Can you work these out from the model? Positions are in its coordinate system, mm. A direction names the side the tool comes from. Give positions to 0.01 mm unless a question says otherwise; leave off trailing zeros. Loops run counter-clockwise (first coordinate to the right, second up) from the corner with the lowest first, then second, coordinate; pieces in that order, holes last. Notation, with made-up numbers: (36, 49) - (56, 49) arc R20 ccw to (56, 85) - close; hole circle Ø3 at (7, 66). An arc over 180 degrees is marked (long way). Write item = value, one per line.
from build123d import *

# Parameters (mm, degrees)
SKETCH_2_R          = 13
EXTRUDE_1_DEPTH     = 1.1
CUT_EXTRUDE_1_REACH = 21.053
SKETCH_3_R          = 7.5


with BuildPart() as part:
    # 草图1 → 旋转1 (revolve)
    with BuildSketch(Plane(origin=(0, 0, 0), x_dir=(-1, 0, 0), z_dir=(0, 0, -1)), mode=Mode.PRIVATE) as revolve_1_sk:
        with BuildLine():
            Line((-11.7, 0), (-7.8, 0))
            Line((-7.8, 0), (-7.5, 0))
            Line((-7.5, 0), (-7.5, 0.3))
            Line((-7.5, 0.3), (-7.5, 4.7))
            ThreePointArc((-7.5, 4.7), (-7.587867966, 4.912132034), (-7.8, 5))
            Line((-7.8, 5), (-11.7, 5))
            ThreePointArc((-11.7, 5), (-11.912132034, 4.912132034), (-12, 4.7))
            Line((-12, 4.7), (-12, 0.3))
            Line((-12, 0.3), (-12, 0))
            Line((-12, 0), (-11.7, 0))
        make_face()
    revolve(revolve_1_sk.sketch.rotate(Axis((0, -0.001250002, 0), (0, 1, 0)), 270), axis=Axis((0, -0.001250002, 0), (0, 1, 0)))

    # 草图2 → 凸台-拉伸1 (add)
    with BuildSketch(Plane.XZ):
        with Locations(Location((0, 0, 0), (0, 0, 270))):
            Circle(SKETCH_2_R)
    extrude(amount=EXTRUDE_1_DEPTH)

    # 草图3 → 切除-拉伸1 (cut, up to next)
    with BuildSketch(Plane(origin=(0, 0, 0), x_dir=(1, 0, 0), z_dir=(0, 1, 0)), mode=Mode.PRIVATE) as cut_extrude_1_sk1:
        with Locations(Location((0, 0, 0), (0, 0, 270))):
            Circle(SKETCH_3_R)
    cut_extrude_1_tool1 = extrude(cut_extrude_1_sk1.sketch, amount=-CUT_EXTRUDE_1_REACH, mode=Mode.PRIVATE) & part.part
    add(cut_extrude_1_tool1.solids().sort_by_distance((0, 0, 0))[0], mode=Mode.SUBTRACT)


solid = part.part
Q1. I need wall thicknesses on L1, parallel to X at y = 2.35, z = 0; L2, parallel to Y at x = 11, z = 6.75. Which ranges of each line are inside material? Lowest first, please.
Output:
L1 = -12 to -7.5, 7.5 to 12
L2 = -1.1 to 0
Q2. Imagine slicing it at A-A, the plane z = 0. Write out the boundary of the cut face in (x, y).
Output:
outline = (-13, -1.1) - (-7.5, -1.1) - (-7.5, 4.7) arc R0.3 ccw to (-7.8, 5) - (-11.7, 5) arc R0.3 ccw to (-12, 4.7) - (-12, 0) - (-13, 0) - close; (7.5, -1.1) - (13, -1.1) - (13, 0) - (12, 0) - (12, 4.7) arc R0.3 ccw to (11.7, 5) - (7.8, 5) arc R0.3 ccw to (7.5, 4.7) - close
Q3. Imagine slicing it at B-B, the plane x = 0. Write out the boundary of the cut face in (y, z).
Output:
outline = (-1.1, -13) - (0, -13) - (0, -12) - (4.7, -12) arc R0.3 ccw to (5, -11.7) - (5, -7.8) arc R0.3 ccw to (4.7, -7.5) - (-1.1, -7.5) - close; (-1.1, 7.5) - (4.7, 7.5) arc R0.3 ccw to (5, 7.8) - (5, 11.7) arc R0.3 ccw to (4.7, 12) - (0, 12) - (0, 13) - (-1.1, 13) - close
Q4. We'd pull the mould along X, two halves only. Please class faces 3 (the cylindrical face through (0.33, 1.841, -7.493)), 4 (the flat face through (-6, -1.1, -6)), 5 (the cylindrical face through (3.604, 2.317, 11.446)): released by +X, released by -X, zero draft, split by the parting line, or undercut.
Output:
face_3 = undercut
face_4 = zero draft
face_5 = split by the parting line
Q5. Which directions (+Z, -Z, +X, -X, +Y, -Y) give clear straight access to the entire face, cutting with the end or side of a thin tool? Please do faces 1 (the flat face through (-9, 0, -9)), 2 (the cylindrical face through (-7.91, -0.542, 10.316)).
Output:
face_1 = +Y
face_2 = +Y, -Y
Q6. For pin 1 (2 mm diameter, centred on y = 1.5, z = -5.5, fed in from -X); pin 2 (3 mm diameter, centred on x = -3.5, y = 3, fed in from -Z); pin 3 (9 mm diameter, centred on x = 0, z = 0, fed in from -Y); pin 4 (1 mm diameter, centred on x = 3.5, y = 3.5, fed in from +Z), each with a flat end and sliding along its axis, tell me the tip position at first contact or that it passes through.
Output:
pin_1 = -11.12
pin_2 = -11.83
pin_3 = through
pin_4 = 11.62
Q7. Imagine slicing it at C-C, the plane y = 1.25. Write out the boundary of the cut face in (x, z).
Output:
outline = circle Ø24 at (0, 0); hole circle Ø15 at (0, 0)
